Could you check a few things on this drawing? It's one solid part, dimensions in mm from its lowest x, y, z. A direction names the side the tool comes from. Round coordinates to 2 decimals unless told otherwise and drop trailing zeros. Answer in a Markdown table with one row per item. Add a question column.
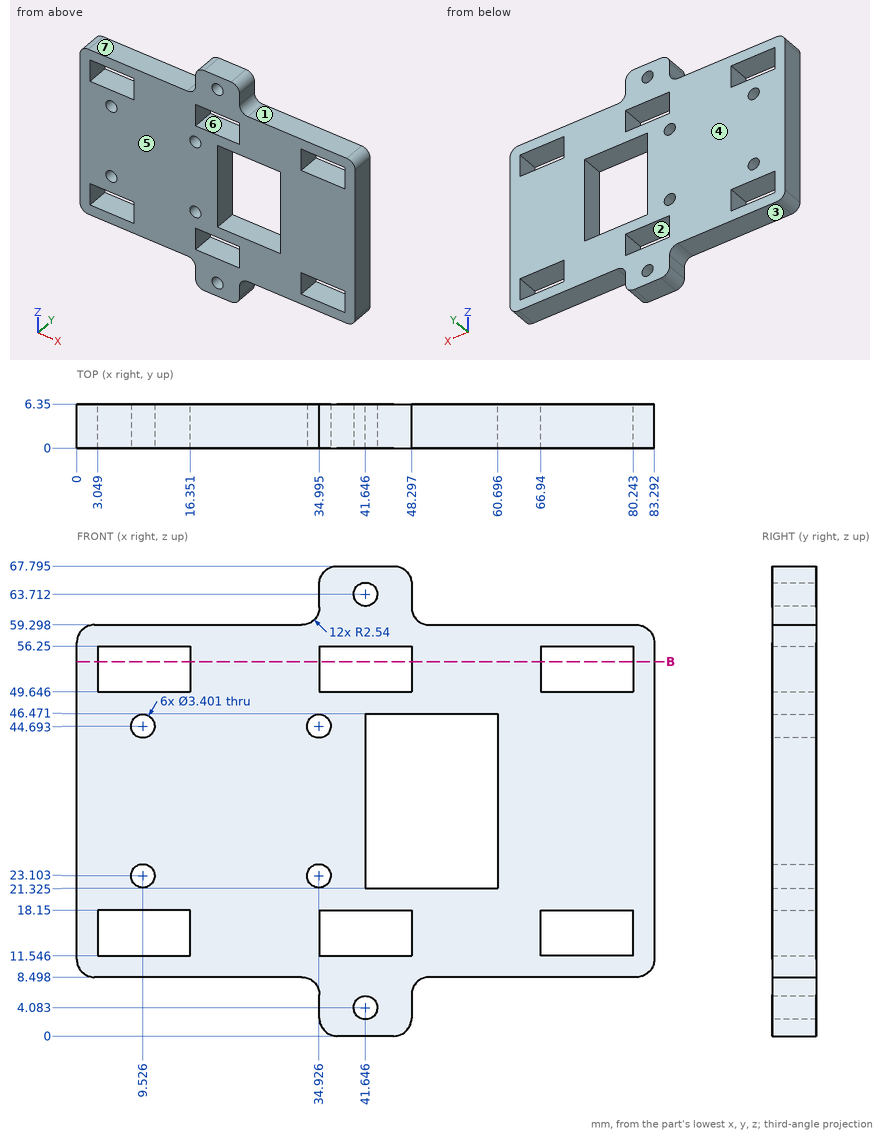
(1) For P1, Ø2, axis at x = 69, y = 0.5, coming from the +Z side; P2, Ø3, axis at x = 41.65, z = 63.71, coming from the -Y side; P3, Ø1.5, axis at y = 1, z = 58.5, coming from the -X side; P4, Ø2, axis at x = 59.5, y = 3, coming from the -Z side, each with a flat end and sliding along its axis, tell me the tip position at first contact or that it passes through.
(2) If we mould it in two halves opening along X, with no side actions, what happens to the marked faces 6 and 7? For each: pulls with the +X half, pulls with the -X half, needs draft (parallel to the pull), parting line crosses it, or undercut.
(3) On a 3-axis mill with a long thin cutter (end or side, diameter ignored), from which of +Z, -Z, +X, -X, +Y, -Y can I reach the whole of each face in a straight line? I mean the marked faces 1, 2, 3, 4 and 5. Say none if no direction works.
(4) Suppose I cut it at B-B, the plane z = 54. State how many separate pieces and enclosed holes the cut face has.
(5) I need wall thicknesses on L1, parallel to Z at x = 58, y = 3.5 (1 decimal); L2, parallel to X at y = 4.5, z = 18 (1 decimal); L3, parallel to X at y = 0.5, z = 41.5 (1 decimal). Which ranges of each line are inside material? Lowest first, please.
Response:
| question | item | result |
|---|---|---|
| 1 | P1 | z = 59.3 |
| 1 | P2 | through |
| 1 | P3 | x = 0.2 |
| 1 | P4 | z = 8.5 |
| 2 | face 6 | undercut |
| 2 | face 7 | needs draft |
| 3 | face 1 | +Z, +X, +Y, -Y |
| 3 | face 2 | +Y, -Y |
| 3 | face 3 | -Z, -X, +Y, -Y |
| 3 | face 4 | +Z, -Z, +X, -X, +Y |
| 3 | face 5 | +Z, -Z, +X, -X, -Y |
| 4 | separate pieces | 4 |
| 4 | enclosed holes | 0 |
| 5 | L1 | 8.5 to 21.3, 46.5 to 59.3 |
| 5 | L2 | 0 to 3, 16.4 to 35, 48.3 to 66.9, 80.2 to 83.3 |
| 5 | L3 | 0 to 41.6, 60.7 to 83.3 |
